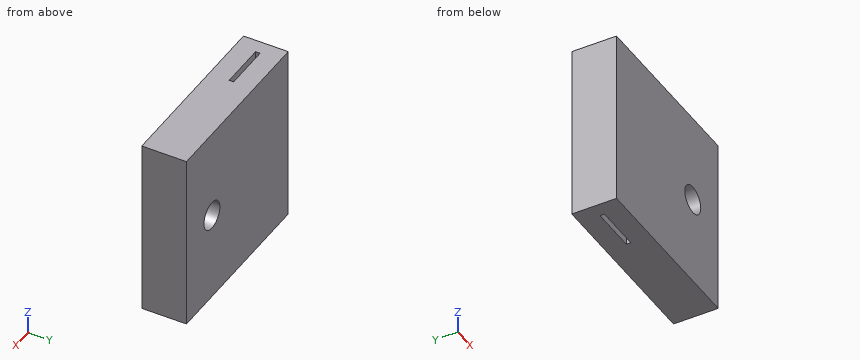
from build123d import *

# Parameters (mm, degrees)
F0_R     = 1.984375
F1_DEPTH = 6.35
F2_W     = 6.604
F2_H     = 0.3175
F3_DEPTH = 76.2


with BuildPart() as f1:
    # F0 (on Front) → F1 (new body)
    with BuildSketch(Plane.XZ):
        Polygon((0, 12.7), (0, 0), (25.4, 0), (25.4, 25.4), (0, 25.4), align=None)
        with Locations((19.05, 12.7)):
            Circle(F0_R, mode=Mode.SUBTRACT)
    extrude(amount=F1_DEPTH)

    # F2 (on face) → F3 (cut)
    with BuildSketch(Plane(origin=(0, 0, 0), x_dir=(1, 0, 0), z_dir=(0, 0, -1))):
        with Locations((5.300516, 3.33375)):
            Rectangle(F2_W, F2_H)
        with Locations((5.300516, 3.01625)):
            Rectangle(F2_W, F2_H)
    extrude(amount=-F3_DEPTH, mode=Mode.SUBTRACT)


solid = f1.part
Model file for the job. Use its own axes, mm. Give positions to 0.01 mm unless a question says otherwise; leave off trailing zeros. Loops run counter-clockwise (first coordinate to the right, second up) from the corner with the lowest first, then second, coordinate; pieces in that order, holes last. Notation, with made-up numbers: (19, -1) - (69, -1) arc R30 ccw to (69, 38) - close; hole circle Ø3 at (1.25, 11). An arc over 180 degrees is marked (long way). Use one line per item in the form item = value.
(1) Cut at C-C (y = -1.5). Give the cut face in (x, z).
Determined:
outline = (0, 0) - (25.4, 0) - (25.4, 25.4) - (0, 25.4) - close; hole circle Ø3.97 at (19.05, 12.7)
(2) Cut at D-D (z = 17.75). Give the cut face in (x, y), then the cut area to 3 significant figures.
Determined:
outline = (0, -6.35) - (25.4, -6.35) - (25.4, 0) - (0, 0) - close; hole (2, -3.49) - (8.6, -3.49) - (8.6, -2.86) - (2, -2.86) - close
area = 157 mm^2
(3) Drill centre lines: L1, parallel to Y at x = 4.5, z = 11.5; L2, parallel to Z at x = 19.05, y = -4.75; L3, parallel to X at y = -3.25, z = 23.5. Where is each one in solid material? Low to high.
Determined:
L1 = -6.35 to -3.49, -2.86 to 0
L2 = 0 to 10.72, 14.68 to 25.4
L3 = 0 to 2, 8.6 to 25.4
(4) Cut at B-B (x = 19.05). Give the cut face in (y, z).
Determined:
outline = (-6.35, 0) - (0, 0) - (0, 10.72) - (-6.35, 10.72) - close; (-6.35, 14.68) - (0, 14.68) - (0, 25.4) - (-6.35, 25.4) - close
(5) Cut at A-A (z = 12.7). Give the cut face in (x, y).
Determined:
outline = (0, -6.35) - (17.07, -6.35) - (17.07, 0) - (0, 0) - close; (21.03, -6.35) - (25.4, -6.35) - (25.4, 0) - (21.03, 0) - close; hole (2, -3.49) - (8.6, -3.49) - (8.6, -2.86) - (2, -2.86) - close
